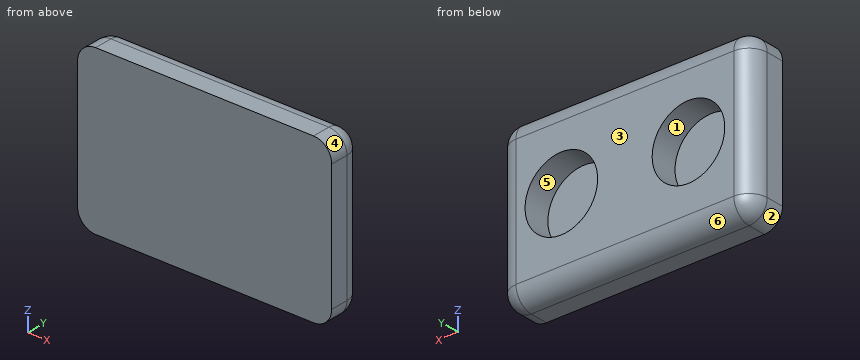
from build123d import *

# Parameters (mm, degrees)
SKETCH1_W           = 140
SKETCH1_H           = 90
BOSS_EXTRUDE1_DEPTH = 20
SKETCH2_R           = 20
CUT_EXTRUDE1_DEPTH  = 15
FILLET1_R           = 10
FILLET2_R           = 10


with BuildPart() as part:
    # Sketch1 → Boss-Extrude1 (new body)
    with BuildSketch(Plane(origin=(0, 0, 0), x_dir=(1, 0, 0), z_dir=(0, 1, 0))):
        Rectangle(SKETCH1_W, SKETCH1_H)
    extrude(amount=BOSS_EXTRUDE1_DEPTH)

    # Sketch2 → Cut-Extrude1 (cut)
    with BuildSketch(Plane(origin=(0, 20, 0), x_dir=(1, 0, 0), z_dir=(0, 1, 0))):
        with Locations((-35, 0)):
            Circle(SKETCH2_R)
        with Locations((35, 0)):
            Circle(SKETCH2_R)
    extrude(amount=-CUT_EXTRUDE1_DEPTH, mode=Mode.SUBTRACT)

    # Fillet1
    fillet1_edges = [part.edges().sort_by_distance(p)[0] for p in [
        (-70, 10, -45),
        (70, 10, -45),
        (70, 10, 45),
        (-70, 10, 45),
    ]]
    fillet(fillet1_edges, radius=FILLET1_R)

    # Fillet2
    fillet2_edges = [part.edges().sort_by_distance(p)[0] for p in [
        (70, 20, 0),
        (0, 20, 45),
        (-70, 20, 0),
        (0, 20, -45),
        (-67.071067812, 20, 42.071067812),
        (-67.071067812, 20, -42.071067812),
        (67.071067812, 20, -42.071067812),
        (67.071067812, 20, 42.071067812),
    ]]
    fillet(fillet2_edges, radius=FILLET2_R)


solid = part.part
Here's how the part is built. I have some questions about the finished solid (model axes, mm). Face numbers are marked on the shaded views. A direction names the side the tool comes from. Coordinates: 2 decimals unless noted, no trailing zeros. Loops run counter-clockwise (first coordinate to the right, second up) from the corner with the lowest first, then second, coordinate; pieces in that order, holes last. Notation, with made-up numbers: (44, 76.25) -> (76, 76.25) arc R34 cw to (76, 112.25) -> close; hole circle Ø9 at (-11, 74.5). An arc over 180 degrees is marked (long way). Use one line per item in the form item = value. Start each with the question number.
(1) Please list where these lines run through material, in increasing order: line 1 along X through (y, z) = (8.25, 0); line 2 along Z through (x, y) = (-36, 7); line 3 along X through (y, z) = (16.5, 0).
(2) Will these pins go through, and if not, where does the flat tip stop? pin 1 (20 mm diameter, centred on x = 33.5, z = 1, fed in from +Y); pin 2 (6 mm diameter, centred on x = 9, y = 16, fed in from +Z).
(3) If we section it at A-A (y = 6.5): Please give me the cut outline in (x, z), then the cut area to 3 significant figures.
(4) We'd pull the mould along X, two halves only. Please class the marked faces 1, 2, 3 and 4: pulls with the +X half, pulls with the -X half, needs draft (parallel to the pull), parting line crosses it, or undercut.
(5) If we section it at D-D (z = 0): Please give me the cut outline in (x, y).
(6) If we section it at B-B (z = 22): Please give me the cut outline in (x, y), then the cut area to 3 significant figures.
(7) On a 3-axis mill with a long thin cutter (end or side, diameter ignored), from which of +Z, -Z, +X, -X, +Y, -Y can I reach the whole of each face in a straight line? I mean the marked faces 5 and 6. Say none if no direction works.
(8) If we section it at C-C (x = -11): Please give me the cut outline in (y, z).
Verdict:
q1.line_1 = -70 to -55, -15 to 15, 55 to 70
q1.line_2 = -45 to -19.97, 19.97 to 45
q1.line_3 = -67.6 to -55, -15 to 15, 55 to 67.6
q2.pin_1 = 5
q2.pin_2 = 44.54
q3.outline = (-70, -35) arc R10 ccw to (-60, -45) -> (60, -45) arc R10 ccw to (70, -35) -> (70, 35) arc R10 ccw to (60, 45) -> (-60, 45) arc R10 ccw to (-70, 35) -> close; hole circle Ø40 at (-35, 0); hole circle Ø40 at (35, 0)
q3.area = 10,000 mm²
q4.face_1 = undercut
q4.face_2 = pulls with the -X half
q4.face_3 = needs draft
q4.face_4 = pulls with the +X half
q5.outline = (-70, 0) -> (70, 0) -> (70, 10) arc R10 ccw to (60, 20) -> (55, 20) -> (55, 5) -> (15, 5) -> (15, 20) -> (-15, 20) -> (-15, 5) -> (-55, 5) -> (-55, 20) -> (-60, 20) arc R10 ccw to (-70, 10) -> close
q6.outline = (-70, 0) -> (70, 0) -> (70, 10) arc R10 ccw to (60, 20) -> (-60, 20) arc R10 ccw to (-70, 10) -> close
q6.area = 2,760 mm²
q7.face_5 = +Y
q7.face_6 = -Z, +X, -X, +Y
q8.outline = (0, -45) -> (10, -45) arc R10 ccw to (20, -35) -> (20, 35) arc R10 ccw to (10, 45) -> (0, 45) -> close
